Can you work these out from the model? Positions are in its coordinate system, mm. A direction names the side the tool comes from. Give positions to 0.01 mm unless a question says otherwise; leave off trailing zeros. Loops run counter-clockwise (first coordinate to the right, second up) from the corner with the lowest first, then second, coordinate; pieces in that order, holes last. Notation, with made-up numbers: (-34.75, 47.25) -> (16.25, 47.25) arc R33 cw to (16.25, 79.25) -> close; hole circle Ø6 at (81, -7.75). An arc over 180 degrees is marked (long way). Return JSON: item names as keys, results as strings. Group by question number.
Q1. Suppose I cut it at D-D, the plane z = -20. Please give me the cut outline in (x, y).
Q2. Thinking about a two-plate mould opening in X: for faces 3 (the cylindrical face through (0.121, 3.448, 17.253)), 4 (the flat face through (-9, 0, 9)), 5 (the cylindrical face through (-40.367, 5.916, -8.964)), which applies, pulls with the +X half, pulls with the -X half, needs draft (parallel to the pull), parting line crosses it, or undercut?
Q3. Suppose I cut it at C-C, the plane y = 2.5. Please give me the cut outline in (x, z), and give its area (3 significant figures).
Q4. Suppose I cut it at A-A, the plane x = 0. Please give me the cut outline in (y, z).
Q5. Will these pins go through, and if not, where does the flat tip stop? pin 1 (4 mm diameter, centred on x = -17, y = 3.5, fed in from +Z); pin 2 (1.5 mm diameter, centred on y = 9.5, z = -21, fed in from -X); pin 3 (4.5 mm diameter, centred on x = 0.5, z = 18, fed in from +Y); pin 4 (14.5 mm diameter, centred on x = 0, z = -20, fed in from +Y).
Q6. Suppose I cut it at B-B, the plane z = 0. Please give me the cut outline in (x, y).
Q7. Which directions (+Z, -Z, +X, -X, +Y, -Y) give clear straight access to the entire face, cutting with the end or side of a thin tool? Please do faces 1 (the flat face through (0, 6.8, -17)), 2 (the flat face through (-9, 12, 9)).
Q8. I need wall thicknesses on line 1 along Z through (x, y) = (5, 1.5); line 2 along Z through (x, y) = (-6, 2.5); line 3 along X through (y, z) = (3.5, 9). Which ranges of each line are inside material? Lowest first, please. Write a range as [from, to].
```python
from build123d import *

# Parameters (mm, degrees)
SKETCH1_R           = 41.35
BOSS_EXTRUDE1_DEPTH = 12
SKETCH2_R           = 2.75
CUT_EXTRUDE1_DEPTH  = 25
SKETCH4_R           = 10.25
CUT_EXTRUDE2_DEPTH  = 25
SKETCH3_R           = 4.5
CUT_EXTRUDE3_DEPTH  = 5.2


with BuildPart() as part:
    # Sketch1 → Boss-Extrude1 (new body)
    with BuildSketch(Plane(origin=(0, 0, 0), x_dir=(1, 0, 0), z_dir=(0, 1, 0))):
        with Locations(Location((0, 0, 0), (0, 0, 270))):
            Circle(SKETCH1_R)
    extrude(amount=BOSS_EXTRUDE1_DEPTH)

    # Sketch2 → Cut-Extrude1 (cut)
    with BuildSketch(Plane(origin=(0, 12, 0), x_dir=(1, 0, 0), z_dir=(0, 1, 0))):
        with Locations(Location((0, 20, 0), (0, 0, 270))):
            Circle(SKETCH2_R)
        with Locations(Location((0, -20, 0), (0, 0, 270))):
            Circle(SKETCH2_R)
    extrude(amount=-CUT_EXTRUDE1_DEPTH, mode=Mode.SUBTRACT)

    # Sketch4 → Cut-Extrude2 (cut)
    with BuildSketch(Plane(origin=(0, 12, 0), x_dir=(1, 0, 0), z_dir=(0, 1, 0))):
        with Locations(Location((0, 0, 0), (0, 0, 270))):
            Circle(SKETCH4_R)
    extrude(amount=-CUT_EXTRUDE2_DEPTH, mode=Mode.SUBTRACT)

    # Sketch3 → Cut-Extrude3 (cut)
    with BuildSketch(Plane(origin=(0, 12, 0), x_dir=(1, 0, 0), z_dir=(0, 1, 0))):
        with Locations(Location((0, 20, 0), (0, 0, 270))):
            Circle(SKETCH3_R)
        with Locations(Location((0, -20, 0), (0, 0, 270))):
            Circle(SKETCH3_R)
    extrude(amount=-CUT_EXTRUDE3_DEPTH, mode=Mode.SUBTRACT)


solid = part.part
```
Ans:
{
 "1": {"outline": "(-36.19, 0) -> (-2.75, 0) -> (-2.75, 6.8) -> (-4.5, 6.8) -> (-4.5, 12) -> (-36.19, 12) -> close; (2.75, 0) -> (36.19, 0) -> (36.19, 12) -> (4.5, 12) -> (4.5, 6.8) -> (2.75, 6.8) -> close"},
 "2": {"face 3": "undercut", "face 4": "needs draft", "face 5": "parting line crosses it"},
 "3": {"outline": "circle Ø82.7 at (0, 0); hole circle Ø20.5 at (0, 0); hole circle Ø5.5 at (0, -20); hole circle Ø5.5 at (0, 20)", "area": "4,990 mm^2"},
 "4": {"outline": "(0, -41.35) -> (12, -41.35) -> (12, -24.5) -> (6.8, -24.5) -> (6.8, -22.75) -> (0, -22.75) -> close; (0, -17.25) -> (6.8, -17.25) -> (6.8, -15.5) -> (12, -15.5) -> (12, -10.25) -> (0, -10.25) -> close; (0, 10.25) -> (12, 10.25) -> (12, 15.5) -> (6.8, 15.5) -> (6.8, 17.25) -> (0, 17.25) -> close; (0, 22.75) -> (6.8, 22.75) -> (6.8, 24.5) -> (12, 24.5) -> (12, 41.35) -> (0, 41.35) -> close"},
 "5": {"pin 1": "stops at z = 38.53", "pin 2": "stops at x = -36.05", "pin 3": "stops at y = 6.8", "pin 4": "stops at y = 12"},
 "6": {"outline": "(-41.35, 0) -> (-10.25, 0) -> (-10.25, 12) -> (-41.35, 12) -> close; (10.25, 0) -> (41.35, 0) -> (41.35, 12) -> (10.25, 12) -> close"},
 "7": {"face 1": "+Y", "face 2": "+Z, -Z, +X, -X, +Y"},
 "8": {"line 1": "z = [-41.05, -8.95], [8.95, 41.05]", "line 2": "z = [-40.91, -8.31], [8.31, 40.91]", "line 3": "x = [-40.36, -4.91], [4.91, 40.36]"}
}
